```python
from build123d import *

# Parameters (mm, degrees)
SKETCH1_R               = 3.125
BOSS_EXTRUDE1_DEPTH     = 19
CUT_EXTRUDE1_DEPTH      = 43.878318603
CUT_EXTRUDE1_DEPTH_BACK = 43.878318603
CUT_EXTRUDE2_START      = -19
CUT_EXTRUDE2_DEPTH      = 4
FILLET2_R               = 3
CUT_EXTRUDE6_DEPTH      = 12.5
CHAMFER1_SIZE           = 2


with BuildPart() as part:
    # Sketch1 → Boss-Extrude1 (new, symmetric)
    # profile 1 of 2: a face of its own
    with BuildSketch(Plane(origin=(0, 0, 0), x_dir=(0, 0, -1), z_dir=(1, 0, 0))):
        with BuildLine():
            ThreePointArc((-26.125, -11), (-24.331029035, -15.331029035), (-20, -17.125))
            Line((-20, -17.125), (29.090970785, -17.125))
            Line((29.090970785, -17.125), (29.090970785, 25.125))
            Line((29.090970785, 25.125), (-3, 25.125))
            ThreePointArc((-3, 25.125), (-9.125, 19), (-3, 12.875))
            Line((-3, 12.875), (9, 12.875))
            ThreePointArc((9, 12.875), (12.535533906, 11.410533906), (14, 7.875))
            Line((14, 7.875), (14, -2.125))
            ThreePointArc((14, -2.125), (13.249270274, -4.760090537), (11.222519145, -6.603884755))
            ThreePointArc((11.222519145, -6.603884755), (-0.005385096, -9.209195056), (-11.208778717, -6.500422867))
            ThreePointArc((-11.208778717, -6.500422867), (-14.508485787, -5.287014241), (-18, -4.875))
            Line((-18, -4.875), (-20, -4.875))
            Line((-20, -4.875), (-26.125, -11))
        make_face()
        with Locations((-20, -11)):
            Circle(SKETCH1_R, mode=Mode.SUBTRACT)
        with BuildLine():
            ThreePointArc((16.391055046, 3.279816514), (18.102037858, 7.993207141), (22.125, 5))
            ThreePointArc((22.125, 5), (21.993207141, 4.102037858), (21.608944954, 3.279816514))
            ThreePointArc((21.608944954, 3.279816514), (20.625, 0), (21.608944954, -3.279816514))
            ThreePointArc((21.608944954, -3.279816514), (21.993207141, -4.102037858), (22.125, -5))
            ThreePointArc((22.125, -5), (18.102037858, -7.993207141), (16.391055046, -3.279816514))
            ThreePointArc((16.391055046, -3.279816514), (17.375, 0), (16.391055046, 3.279816514))
        make_face(mode=Mode.SUBTRACT)
        with BuildLine():
            ThreePointArc((-0.945205479, 16.645547945), (-6.125, 19), (-0.945205479, 21.354452055))
            ThreePointArc((-0.945205479, 21.354452055), (1, 20.625), (2.945205479, 21.354452055))
            ThreePointArc((2.945205479, 21.354452055), (6.293134201, 21.844895242), (8.125, 19))
            ThreePointArc((8.125, 19), (6.293134201, 16.155104758), (2.945205479, 16.645547945))
            ThreePointArc((2.945205479, 16.645547945), (1, 17.375), (-0.945205479, 16.645547945))
        make_face(mode=Mode.SUBTRACT)
    # profile 2 of 2: a face of its own
    with BuildSketch(Plane(origin=(0, 0, 0), x_dir=(0, 0, -1), z_dir=(1, 0, 0))):
        with BuildLine():
            ThreePointArc((-20, -4.875), (-24.331029035, -6.668970965), (-26.125, -11))
            Line((-26.125, -11), (-20, -4.875))
        make_face()
    extrude(amount=BOSS_EXTRUDE1_DEPTH, both=True)

    # Sketch2 → Cut-Extrude1 (cut, two sides: drawn at the far end of the back side and taken through both)
    with BuildSketch(Plane(origin=(0, 0, 0), x_dir=(0, 0, -1), z_dir=(1, 0, 0)).offset(-CUT_EXTRUDE1_DEPTH_BACK)):
        with BuildLine():
            Line((-12.02081528, 13.62081528), (-15.02081528, 13.62081528))
            ThreePointArc((-15.02081528, 13.62081528), (-16.62081528, 12.02081528), (-15.02081528, 10.42081528))
            Line((-15.02081528, 10.42081528), (-12.02081528, 10.42081528))
            ThreePointArc((-12.02081528, 10.42081528), (-10.42081528, 12.02081528), (-12.02081528, 13.62081528))
        make_face()
        with BuildLine():
            Line((12.02081528, 13.62081528), (9.02081528, 13.62081528))
            ThreePointArc((9.02081528, 13.62081528), (7.42081528, 12.02081528), (9.02081528, 10.42081528))
            Line((9.02081528, 10.42081528), (12.02081528, 10.42081528))
            ThreePointArc((12.02081528, 10.42081528), (13.62081528, 12.02081528), (12.02081528, 13.62081528))
        make_face()
        with BuildLine():
            Line((12.02081528, -10.42081528), (9.02081528, -10.42081528))
            ThreePointArc((9.02081528, -10.42081528), (7.42081528, -12.02081528), (9.02081528, -13.62081528))
            Line((9.02081528, -13.62081528), (12.02081528, -13.62081528))
            ThreePointArc((12.02081528, -13.62081528), (13.62081528, -12.02081528), (12.02081528, -10.42081528))
        make_face()
        with BuildLine():
            Line((-12.02081528, -10.42081528), (-15.02081528, -10.42081528))
            ThreePointArc((-15.02081528, -10.42081528), (-16.62081528, -12.02081528), (-15.02081528, -13.62081528))
            Line((-15.02081528, -13.62081528), (-12.02081528, -13.62081528))
            ThreePointArc((-12.02081528, -13.62081528), (-10.42081528, -12.02081528), (-12.02081528, -10.42081528))
        make_face()
    extrude(amount=CUT_EXTRUDE1_DEPTH + CUT_EXTRUDE1_DEPTH_BACK, mode=Mode.SUBTRACT)

    # Sketch2<3> → Cut-Extrude2 (cut)
    # profile 1 of 4: a face of its own
    with BuildSketch(Plane(origin=(0, 0, 0), x_dir=(0, 0, -1), z_dir=(1, 0, 0)).offset(CUT_EXTRUDE2_START)):
        with BuildLine():
            Line((-12.02081528, 9.02081528), (-15.02081528, 9.02081528))
            ThreePointArc((-15.02081528, 9.02081528), (-18.02081528, 12.02081528), (-15.02081528, 15.02081528))
            Line((-15.02081528, 15.02081528), (-12.02081528, 15.02081528))
            ThreePointArc((-12.02081528, 15.02081528), (-9.02081528, 12.02081528), (-12.02081528, 9.02081528))
        make_face()
        with BuildLine():
            Line((-12.02081528, 10.42081528), (-15.02081528, 10.42081528))
            ThreePointArc((-15.02081528, 10.42081528), (-16.62081528, 12.02081528), (-15.02081528, 13.62081528))
            Line((-15.02081528, 13.62081528), (-12.02081528, 13.62081528))
            ThreePointArc((-12.02081528, 13.62081528), (-10.42081528, 12.02081528), (-12.02081528, 10.42081528))
        make_face(mode=Mode.SUBTRACT)
    # profile 2 of 4: a face of its own
    with BuildSketch(Plane(origin=(0, 0, 0), x_dir=(0, 0, -1), z_dir=(1, 0, 0)).offset(CUT_EXTRUDE2_START)):
        with BuildLine():
            Line((-12.02081528, -15.02081528), (-15.02081528, -15.02081528))
            ThreePointArc((-15.02081528, -15.02081528), (-18.02081528, -12.02081528), (-15.02081528, -9.02081528))
            Line((-15.02081528, -9.02081528), (-12.02081528, -9.02081528))
            ThreePointArc((-12.02081528, -9.02081528), (-9.02081528, -12.02081528), (-12.02081528, -15.02081528))
        make_face()
        with BuildLine():
            Line((-12.02081528, -13.62081528), (-15.02081528, -13.62081528))
            ThreePointArc((-15.02081528, -13.62081528), (-16.62081528, -12.02081528), (-15.02081528, -10.42081528))
            Line((-15.02081528, -10.42081528), (-12.02081528, -10.42081528))
            ThreePointArc((-12.02081528, -10.42081528), (-10.42081528, -12.02081528), (-12.02081528, -13.62081528))
        make_face(mode=Mode.SUBTRACT)
    # profile 3 of 4: a face of its own
    with BuildSketch(Plane(origin=(0, 0, 0), x_dir=(0, 0, -1), z_dir=(1, 0, 0)).offset(CUT_EXTRUDE2_START)):
        with BuildLine():
            Line((12.02081528, -15.02081528), (9.02081528, -15.02081528))
            ThreePointArc((9.02081528, -15.02081528), (6.02081528, -12.02081528), (9.02081528, -9.02081528))
            Line((9.02081528, -9.02081528), (12.02081528, -9.02081528))
            ThreePointArc((12.02081528, -9.02081528), (15.02081528, -12.02081528), (12.02081528, -15.02081528))
        make_face()
        with BuildLine():
            Line((12.02081528, -13.62081528), (9.02081528, -13.62081528))
            ThreePointArc((9.02081528, -13.62081528), (7.42081528, -12.02081528), (9.02081528, -10.42081528))
            Line((9.02081528, -10.42081528), (12.02081528, -10.42081528))
            ThreePointArc((12.02081528, -10.42081528), (13.62081528, -12.02081528), (12.02081528, -13.62081528))
        make_face(mode=Mode.SUBTRACT)
    # profile 4 of 4: a face of its own
    with BuildSketch(Plane(origin=(0, 0, 0), x_dir=(0, 0, -1), z_dir=(1, 0, 0)).offset(CUT_EXTRUDE2_START)):
        with BuildLine():
            Line((12.02081528, 9.02081528), (9.02081528, 9.02081528))
            ThreePointArc((9.02081528, 9.02081528), (6.02081528, 12.02081528), (9.02081528, 15.02081528))
            Line((9.02081528, 15.02081528), (12.02081528, 15.02081528))
            ThreePointArc((12.02081528, 15.02081528), (15.02081528, 12.02081528), (12.02081528, 9.02081528))
        make_face()
        with BuildLine():
            Line((12.02081528, 10.42081528), (9.02081528, 10.42081528))
            ThreePointArc((9.02081528, 10.42081528), (7.42081528, 12.02081528), (9.02081528, 13.62081528))
            Line((9.02081528, 13.62081528), (12.02081528, 13.62081528))
            ThreePointArc((12.02081528, 13.62081528), (13.62081528, 12.02081528), (12.02081528, 10.42081528))
        make_face(mode=Mode.SUBTRACT)
    extrude(amount=CUT_EXTRUDE2_DEPTH, mode=Mode.SUBTRACT)

    # Fillet2
    fillet2_edges = [part.edges().sort_by_distance(p)[0] for p in [
        (2, 10.800069224, -13.055116526),
        (-17, 9.543812481, -13.713285998),
        (-17, 12.875, -6.144990448),
        (-17, -13.199102102, 17.779735389),
        (-17, -9.851965995, 17.093517087),
        (2, 12.875, -7.667904173),
    ]]
    fillet(fillet2_edges, radius=FILLET2_R)

    # Sketch1<4> → Cut-Extrude6 (cut, symmetric)
    with BuildSketch(Plane(origin=(0, 0, 0), x_dir=(0, 0, -1), z_dir=(1, 0, 0))):
        with BuildLine():
            ThreePointArc((-20, -4.875), (-24.331029035, -6.668970965), (-26.125, -11))
            Line((-26.125, -11), (-20, -4.875))
        make_face()
    extrude(amount=CUT_EXTRUDE6_DEPTH, both=True, mode=Mode.SUBTRACT)

    # Chamfer1
    # the kernel refuses this chamfer: 2 mm, written as the material it adds along each edge
    with BuildSketch(Plane(origin=(12.5, -14.63690896, 29.76190896), x_dir=(-0.9996219169112968, -0.01944252080601336, -0.019442520806013355), z_dir=(0, 0.7071067811865475, -0.7071067811865476))) as chamfer1_piece_1_section:
        Polygon((CHAMFER1_SIZE * 0.999621916911, CHAMFER1_SIZE * 0.0274958766106), (-CHAMFER1_SIZE * 0.0274958766106, CHAMFER1_SIZE * 0.999621916911), (0, 0), align=None)
    chamfer1_piece_1 = extrude(amount=18.948790021, mode=Mode.PRIVATE)
    chamfer1_piece_1 = chamfer1_piece_1 & Plane(origin=(11.776447372, -11, 20), x_dir=(0, 0, 1), z_dir=(1, 0, 0)) * Cylinder(6.125, 46, mode=Mode.PRIVATE)
    add(chamfer1_piece_1)
    with BuildSketch(Plane(origin=(-12.5, -14.63690896, 29.76190896), x_dir=(0.9996219169112968, -0.01944252080601336, -0.019442520806013355), z_dir=(0, 0.7071067811865475, -0.7071067811865476))) as chamfer1_piece_2_section:
        Polygon((CHAMFER1_SIZE * 0.999621916911, -CHAMFER1_SIZE * 0.0274958766106), (-CHAMFER1_SIZE * 0.0274958766106, -CHAMFER1_SIZE * 0.999621916911), (0, 0), align=None)
    chamfer1_piece_2 = extrude(amount=18.948790021, mode=Mode.PRIVATE)
    chamfer1_piece_2 = chamfer1_piece_2 & Plane(origin=(-11.776447372, -11, 20), x_dir=(0, 0, 1), z_dir=(1, 0, 0)) * Cylinder(6.125, 46, mode=Mode.PRIVATE)
    add(chamfer1_piece_2)


solid = part.part
```
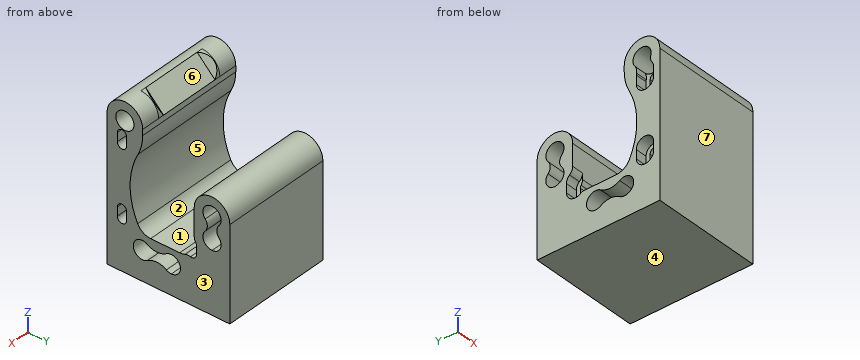
Work out the finished part from the listing and answer in its coordinate system (mm). Face numbers are marked on the shaded views. A direction names the side the tool comes from. Round coordinates to 2 decimals unless told otherwise and drop trailing zeros. Write each loop counter-clockwise with the first axis right and the second up, starting at its lowest first coordinate (ties: lowest second). Pieces come first, ordered by that corner, then holes.
1) A cutting plane is placed at D-D on x = 2. Give the number of separate pieces and of enclosed holes in the cut face, and give its area (3 significant figures).
2) Which of the six approach directions +Z, -Z, +X, -X, +Y, -Y give full straight-line access (tool end or side, diameter ignored) to the marked faces 1, 2 and 3?
3) Consider probe 1 along Z at (x, y) = (2, 19) (3 decimals); probe 2 along Y at (x, z) = (6.5, -2) (3 decimals); probe 3 along Y at (x, z) = (-13, 20) (3 decimals). Determine where each line is inside the solid, lowest interval first.
4) A cutting plane is placed at B-B on y = 0.5. Determine the outline of the cut face in (x, z), and give its area (3 significant figures).
5) Flat-ended cylindrical pins translate along their axes: P1, Ø1.5, axis at y = -5, z = 9.5, coming from the +X side; P2, Ø3.5, axis at x = 3.5, z = 14, coming from the +Y side; P3, Ø4, axis at x = 11.5, y = -7.5, coming from the +Z side; P4, Ø11, axis at x = 6, y = 2.5, coming from the +Z side. Find the tip coordinate at first contact, or state that the pin passes through.
6) A cutting plane is placed at C-C on z = 13. Determine the outline of the cut face in (x, y) (3 decimals), and give its area (3 significant figures).
7) A cutting plane is placed at A-A on z = -19. Determine the outline of the cut face in (x, y) (3 decimals).
8) Determine the mould class of the marked faces 4, 5, 6 and 7 for opening direction Y: pulls with the +Y half, pulls with the -Y half, needs draft (parallel to the pull), parting line crosses it, or undercut.
Entries:
1. separate pieces: 1
1. enclosed holes: 5
1. area: 1,070 mm2
2. face 1: +Z, +X, -X
2. face 2: +X, -X
2. face 3: +Z, -Z, +X, +Y, -Y
3. probe 1: z = -29.091 to -8.125, 6.125 to 9.125
3. probe 2: y = -17.125 to -9.138, 12.875 to 17.201, 20.799 to 25.125
3. probe 3: y = -17.125 to -14.125, -7.875 to -4.875
4. outline: (-19, -29.09) - (19, -29.09) - (19, -20.65) - (-19, -20.65) - close; (-19, -17.35) - (19, -17.35) - (19, -14) - (-19, -14) - close
4. area: 448 mm2
5. P1: passes through
5. P2: stops at y = -5.04
5. P3: stops at z = 25.94
5. P4: stops at z = -13.92
6. outline: (-19, -17.125) - (19, -17.125) - (19, -13.621) - (-15, -13.621) - (-15, -15.021) - (-19, -15.021) - close; (-19, -9.021) - (-15, -9.021) - (-15, -10.421) - (19, -10.421) - (19, -5.733) - (-19, -5.733) - close
6. area: 300 mm2
7. outline: (-19, -17.125) - (19, -17.125) - (19, -8.125) - (-19, -8.125) - close; (-19, 8.125) - (19, 8.125) - (19, 25.125) - (-19, 25.125) - close
8. face 4: needs draft
8. face 5: undercut
8. face 6: pulls with the +Y half
8. face 7: pulls with the -Y half
